```python
from build123d import *

# Parameters (mm, degrees)
JOIN1_START         = -4.2
JOIN1_OUTLINE_R     = 5
JOIN1_DEPTH         = 4.2
JOIN1_START_2       = -6.3
JOIN1_2_OUTLINE_R   = 7.5
JOIN1_2_OUTLINE_R_2 = 5
JOIN1_2_DEPTH       = 12
JOIN1_3_OUTLINE_R   = 10
JOIN1_3_OUTLINE_R_2 = 7.5
JOIN1_3_DEPTH       = 2.1
SKETCH1_W           = 3
SKETCH1_H           = 4.738081577
CUT_EXTRUDE1_DEPTH  = 38.271436785
SKETCH2_R           = 1.5
CUT_EXTRUDE2_DEPTH  = 1
CIRPATTERN1_COUNT   = 12
CHAMFER1_SIZE       = 0.2
CHAMFER2_SIZE       = 0.2
CHAMFER3_SIZE       = 0.3


# Read off the part's stored shape, not the designer's step: Join1
with BuildPart() as part:
    # Join1 outline → Join1 (new body)
    with BuildSketch(Plane.XY.offset(JOIN1_START)):
        with BuildLine():
            ThreePointArc((-24.903011866, -2.2), (0, -25), (24.903011866, -2.2))
            Line((24.903011866, -2.2), (11.86423196, -2.2))
            ThreePointArc((11.86423196, -2.2), (9.256550998, -1.233150178), (7.909487973, 1.2))
            ThreePointArc((7.909487973, 1.2), (0, 8), (-7.909487973, 1.2))
            ThreePointArc((-7.909487973, 1.2), (-9.256550998, -1.233150178), (-11.86423196, -2.2))
            Line((-11.86423196, -2.2), (-24.903011866, -2.2))
        make_face()
        Circle(JOIN1_OUTLINE_R, mode=Mode.SUBTRACT)
    extrude(amount=JOIN1_DEPTH)

    # Join1 2 outline → Join1 2 (add)
    with BuildSketch(Plane.XY.offset(JOIN1_START_2)):
        Circle(JOIN1_2_OUTLINE_R)
        Circle(JOIN1_2_OUTLINE_R_2, mode=Mode.SUBTRACT)
    extrude(amount=JOIN1_2_DEPTH)

    # Join1 3 outline → Join1 3 (add)
    with BuildSketch(Plane.XY.offset(JOIN1_START_2)):
        Circle(JOIN1_3_OUTLINE_R)
        Circle(JOIN1_3_OUTLINE_R_2, mode=Mode.SUBTRACT)
    extrude(amount=JOIN1_3_DEPTH)

    # Sketch1 → Cut-Extrude1 (cut, through all)
    with BuildSketch(Plane.XY.offset(5.7)):
        with Locations((0, -4.130959212)):
            Rectangle(SKETCH1_W, SKETCH1_H)
    extrude(amount=-CUT_EXTRUDE1_DEPTH, mode=Mode.SUBTRACT)

    # Sketch2 → Cut-Extrude2 (cut)
    with BuildSketch(Plane(origin=(0, 0, -6.3), x_dir=(-1, 0, 0), z_dir=(0, 0, -1))):
        with Locations((-7.5, 0)):
            Circle(SKETCH2_R)
    cut_extrude2 = extrude(amount=-CUT_EXTRUDE2_DEPTH, mode=Mode.SUBTRACT)

    # CirPattern1: Cut-Extrude2 ×12 about axis
    cirpattern1_axis = Axis((0, 0, 0), (0, 0, 1))
    for i in range(1, CIRPATTERN1_COUNT):
        add(cut_extrude2.rotate(cirpattern1_axis, i * 360 / CIRPATTERN1_COUNT), mode=Mode.SUBTRACT)

    # Chamfer1
    chamfer1_edges = [part.edges().sort_by_distance(p)[0] for p in [
        (0, 5, 5.7),
    ]]
    chamfer(chamfer1_edges, length=CHAMFER1_SIZE)

    # Chamfer2
    chamfer2_edges = [part.edges().sort_by_distance(p)[0] for p in [
        (0, 5, -6.3),
    ]]
    chamfer(chamfer2_edges, length=CHAMFER2_SIZE)

    # Chamfer3
    chamfer3_edges = [part.edges().sort_by_distance(p)[0] for p in [
        (0, -25, 0),
    ]]
    chamfer(chamfer3_edges, length=CHAMFER3_SIZE)


solid = part.part
```
Part model, mm, in its own coordinate system. A direction names the side the tool comes from. Round coordinates to 2 decimals unless told otherwise and drop trailing zeros. Write each loop counter-clockwise with the first axis right and the second up, starting at its lowest first coordinate (ties: lowest second). Pieces come first, ordered by that corner, then holes. Notation, with made-up numbers: M 6.25,61 L 43.25,61 A24 cw 43.25,93 Z; hole C -31,10 d1. An arc over 180 degrees is marked long. One line per question, with ' | ' between items.
(1) Saw through at A-A on x = 0. Write the cut outline in (y, z), then the cut area to 3 significant figures.
Answer key:
outline: M -25,-4.2 L -10,-4.2 L -10,-6.3 L -9,-6.3 L -9,-5.3 L -6.5,-5.3 L -6.5,5.7 L -7.5,5.7 L -7.5,0 L -24.7,0 L -25,-0.3 Z; M 5,-6.1 L 5.2,-6.3 L 6,-6.3 L 6,-5.3 L 9,-5.3 L 9,-6.3 L 10,-6.3 L 10,-4.2 L 8,-4.2 L 8,0 L 7.5,0 L 7.5,5.7 L 5.2,5.7 L 5,5.5 Z | area: 123 mm^2
(2) Saw through at B-B on z = -2. Write the cut outline in (x, y), then the cut area to 3 significant figures.
Answer key:
outline: M -24.9,-2.2 A25 ccw 24.9,-2.2 L 11.86,-2.2 A4 cw 7.91,1.2 A8 ccw -7.91,1.2 A4 cw -11.86,-2.2 Z; hole M -1.5,-6.5 L 1.5,-6.5 L 1.5,-4.77 A5 ccw long -1.5,-4.77 Z | area: 930 mm^2
(3) Saw through at D-D on z = 3.75. Write the cut outline in (x, y).
Answer key:
outline: C 0,0 d15; hole M -1.5,-6.5 L 1.5,-6.5 L 1.5,-4.77 A5 ccw long -1.5,-4.77 Z
(4) Two-plate mould, pull along Y, no slides. Class faces 1 (the face through (-7.493, 0.33, 2.81)), 2 (the face through (5.01, -3.55, -5.81)), 3 (the face through (8, 0, -5.3)), 4 (the face through (-2, -5, 5.7)): released by +Y, released by -Y, zero draft, split by the parting line, or undercut.
Answer key:
face 1: split by the parting line | face 2: undercut | face 3: undercut | face 4: zero draft
(5) 3-axis set-ups, long thin cutter, end or side, ignore diameter. For faces 5 (the face through (0, -8, -5.3)), 6 (the face through (-5.2, -1.4, -6.3)), 7 (the face through (-18, -2.2, -2)): which of +Z, -Z, +X, -X, +Y, -Y reach the whole face in a straight line?
Answer key:
face 5: -Z | face 6: -Z, +X, -X, +Y, -Y | face 7: +Z, -Z, -X, +Y
(6) Saw through at C-C on y = 0. Write the cut outline in (x, z), then the cut area to 3 significant figures.
Answer key:
outline: M -10,-6.3 L -9,-6.3 L -9,-5.3 L -6,-5.3 L -6,-6.3 L -5.2,-6.3 L -5,-6.1 L -5,5.5 L -5.2,5.7 L -7.5,5.7 L -7.5,0 L -8.29,0 L -8.29,-4.2 L -10,-4.2 Z; M 5,-6.1 L 5.2,-6.3 L 6,-6.3 L 6,-5.3 L 9,-5.3 L 9,-6.3 L 10,-6.3 L 10,-4.2 L 8.29,-4.2 L 8.29,0 L 7.5,0 L 7.5,5.7 L 5.2,5.7 L 5,5.5 Z | area: 71.1 mm^2
(7) Pin check, flat tips, straight feed: pin 1 (1.5 mm diameter, centred on x = 17, y = -4, fed in from -Z); pin 2 (2.5 mm diameter, centred on x = -6.5, y = -4.5, fed in from -Z); pin 3 (2 mm diameter, centred on y = -19.5, z = 2, fed in from -X); pin 4 (0.9 mm diameter, centred on y = -5.5, z = 0, fed in from -X). Stop position of each tip, or through.
Answer key:
pin 1: stops at z = -4.2 | pin 2: stops at z = -6.3 | pin 3: passes through | pin 4: stops at x = -24.46
(8) Probe line 1 along X through (y, z) = (-7.5, -5.6); line 2 along X through (y, z) = (3.75, -5.55). List the from-to ranges inside material, lowest first.
Answer key:
line 1: x = -6.61 to -4.86, -2.64 to -1.5, 1.5 to 2.64, 4.86 to 6.61 | line 2: x = -9.27 to -8, -5 to -3.31, 3.31 to 5, 8 to 9.27
